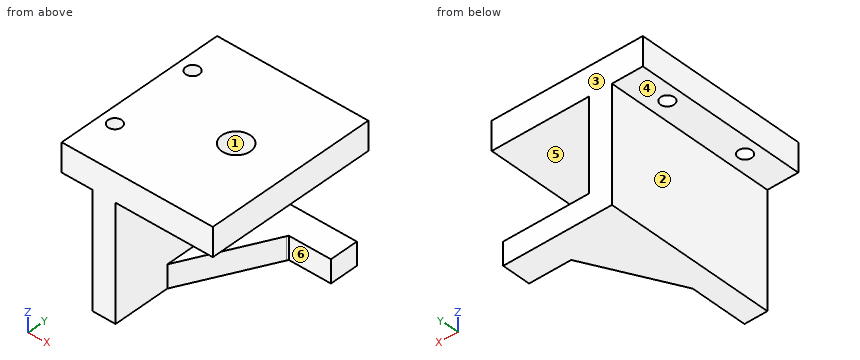
```python
from build123d import *

# Parameters (mm, degrees)
SKETCH2_W           = 6.35
SKETCH2_H           = 38.1
BOSS_EXTRUDE1_DEPTH = 19.05
SKETCH3_R           = 1.5
CUT_EXTRUDE1_DEPTH  = 28.679008291
SKETCH4_W           = 14.478
SKETCH4_H           = 6.35
SKETCH4_W_2         = 9.525
SKETCH4_H_2         = 5.08
BOSS_EXTRUDE2_DEPTH = 38.1
SKETCH5_R           = 3.175
CUT_EXTRUDE2_DEPTH  = 6.35
CUT_EXTRUDE3_DEPTH  = 5.08
BOSS_EXTRUDE3_DEPTH = 5.08


with BuildPart() as part:
    # Sketch2 → Boss-Extrude1 (new body)
    with BuildSketch(Plane(origin=(0, 0, 0), x_dir=(0, 0, -1), z_dir=(1, 0, 0))):
        Rectangle(SKETCH2_W, SKETCH2_H)
    extrude(amount=BOSS_EXTRUDE1_DEPTH)

    # Sketch3 → Cut-Extrude1 (cut, through all)
    with BuildSketch(Plane.XY.offset(3.175)):
        with Locations((3.175, 9.525)):
            Circle(SKETCH3_R)
        with Locations((3.175, -9.525)):
            Circle(SKETCH3_R)
    extrude(amount=-CUT_EXTRUDE1_DEPTH, mode=Mode.SUBTRACT)

    # Sketch4 → Boss-Extrude2 (add)
    with BuildSketch(Plane(origin=(0, 19.05, 0), x_dir=(1, 0, 0), z_dir=(0, 1, 0))):
        with Locations((26.289, 0)):
            Rectangle(SKETCH4_W, SKETCH4_H)
        Polygon((6.858, 3.175), (6.858, -3.175), (19.05, -3.175), (19.05, 3.175), (11.938, 3.175), align=None)
        Polygon((6.858, 28.575), (6.858, 3.175), (11.938, 3.175), (11.938, 23.495), (11.938, 28.575), align=None)
        with Locations((16.7005, 26.035)):
            Rectangle(SKETCH4_W_2, SKETCH4_H_2)
    extrude(amount=-BOSS_EXTRUDE2_DEPTH)

    # Sketch5 → Cut-Extrude2 (cut)
    with BuildSketch(Plane.XY.offset(3.175)):
        with Locations((21.463, 0)):
            Circle(SKETCH5_R)
    extrude(amount=-CUT_EXTRUDE2_DEPTH, mode=Mode.SUBTRACT)

    # Sketch6 → Cut-Extrude3 (cut)
    with BuildSketch(Plane(origin=(0, 0, -28.575), x_dir=(-1, 0, 0), z_dir=(0, 0, -1))):
        Polygon((-21.463, -19.05), (-11.938, -19.05), (-11.938, -6.35), (-21.463, 12.343865065), align=None)
    extrude(amount=-CUT_EXTRUDE3_DEPTH, mode=Mode.SUBTRACT)

    # Sketch6<3> → Boss-Extrude3 (add)
    with BuildSketch(Plane(origin=(0, 0, -28.575), x_dir=(-1, 0, 0), z_dir=(0, 0, -1))):
        Polygon((-21.463, 12.343865065), (-21.463, 19.05), (-30.988, 19.05), (-30.988, 12.7), (-21.644459813, 12.7), align=None)
    extrude(amount=-BOSS_EXTRUDE3_DEPTH)


solid = part.part
```
Read the model definition and answer for the solid it produces. Units are mm, in the model's axes. Face numbers are marked on the shaded views. A direction names the side the tool comes from. Coordinates: 2 decimals unless noted, no trailing zeros. Loops run counter-clockwise (first coordinate to the right, second up) from the corner with the lowest first, then second, coordinate; pieces in that order, holes last.
(1) The part is cut by section C-C (z = -2.5). Determine the outline of the cut face in (x, y) (3 decimals), and give its area (3 significant figures).
Solution:
outline: (0, -19.05) - (33.528, -19.05) - (33.528, 19.05) - (0, 19.05) - close; hole circle Ø3 at (3.175, -9.525); hole circle Ø3 at (3.175, 9.525); hole circle Ø6.35 at (21.463, 0)
area: 1,230 mm2
(2) The part is cut by section A-A (x = 26). Determine the outline of the cut face in (y, z) (3 decimals).
Solution:
outline: (-19.05, -3.175) - (19.05, -3.175) - (19.05, 3.175) - (-19.05, 3.175) - close; (12.7, -28.575) - (19.05, -28.575) - (19.05, -23.495) - (12.7, -23.495) - close
(3) Flat-ended cylindrical pins translate along their axes: pin 1 Ø3 at (y, z) = (14, -19.5) entering from -X; pin 2 Ø8 at (x, y) = (25, 9) entering from -Z (3 decimals); pin 3 Ø5.5 at (x, y) = (3, -7.5) entering from -Z (3 decimals); pin 4 Ø1.5 at (y, z) = (17, -25.5) entering from +X. Find the tip coordinate at first contact, or state that the pin passes through.
Solution:
pin 1: stops at x = 6.86
pin 2: stops at z = -28.575
pin 3: stops at z = -3.175
pin 4: stops at x = 30.99
(4) Consider line 1 along Z through (x, y) = (12.5, 1) (3 decimals); line 2 along Z through (x, y) = (15, -11.5) (3 decimals); line 3 along X through (y, z) = (-3, -23). Determine where each line is inside the solid, lowest interval first.
Solution:
line 1: z = -28.575 to -23.495, -3.175 to 3.175
line 2: z = -3.175 to 3.175
line 3: x = 6.86 to 11.94
(5) The part is cut by section D-D (x = 12.5). Determine the outline of the cut face in (y, z) (3 decimals).
Solution:
outline: (-19.05, -3.175) - (19.05, -3.175) - (19.05, 3.175) - (-19.05, 3.175) - close; (-5.247, -28.575) - (19.05, -28.575) - (19.05, -23.495) - (-5.247, -23.495) - close
(6) A tool of negligible diameter and unlimited length cuts with its end or side. For the marked faces 4, 5 and 6, from which of +Z, -Z, +X, -X, +Y, -Y can it reach the whole face along a straight path? Write none if from no direction.
Solution:
face 4: -Z, -X, +Y, -Y
face 5: +X, +Y, -Y
face 6: -Z, +X, -Y
(7) The part is cut by section B-B (y = -2). Determine the outline of the cut face in (x, z) (3 decimals).
Solution:
outline: (0, -3.175) - (6.858, -3.175) - (6.858, -28.575) - (14.154, -28.575) - (14.154, -23.495) - (11.938, -23.495) - (11.938, -3.175) - (18.997, -3.175) - (18.997, 3.175) - (0, 3.175) - close; (23.929, -3.175) - (33.528, -3.175) - (33.528, 3.175) - (23.929, 3.175) - close
(8) The mould has two halves that part along X. Classify the marked faces 1, 2 and 3: released by +X, released by -X, zero draft, split by the parting line, or undercut.
Solution:
face 1: undercut
face 2: released by -X
face 3: zero draft
